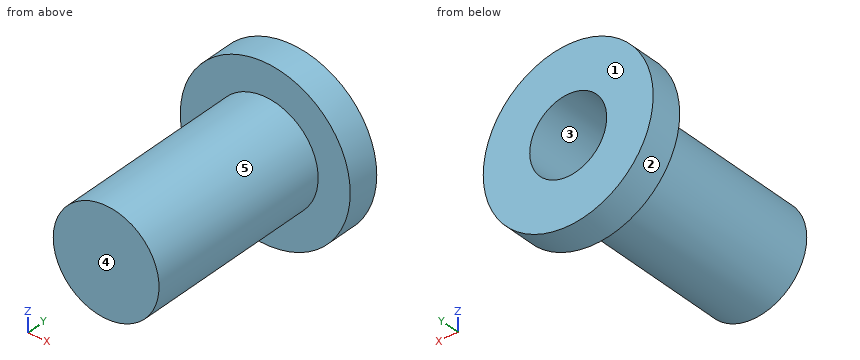
from build123d import *

# Parameters (mm, degrees)
SKETCH3_R          = 1.2
CUT_EXTRUDE1_DEPTH = 5.8


with BuildPart() as part:
    # Sketch2 → Revolve2 (revolve)
    with BuildSketch(Plane.XY):
        Polygon((-1.65, 0), (-1.65, -6), (0, -6), (0, 1), (-2.65, 1), (-2.65, 0), align=None)
    revolve(axis=Axis((0, 2, 0), (0, -1, 0)))

    # Sketch3 → Cut-Extrude1 (cut)
    with BuildSketch(Plane(origin=(0, 1, 0), x_dir=(1, 0, 0), z_dir=(0, 1, 0))):
        Circle(SKETCH3_R)
    extrude(amount=-CUT_EXTRUDE1_DEPTH, mode=Mode.SUBTRACT)


solid = part.part
Build history of the part. All positions in model axes, mm. Face numbers are marked on the shaded views. A direction names the side the tool comes from. Give positions to 0.01 mm unless a question says otherwise; leave off trailing zeros. Loops run counter-clockwise (first coordinate to the right, second up) from the corner with the lowest first, then second, coordinate; pieces in that order, holes last. Notation, with made-up numbers: (-23, 86.25) - (-10, 86.25) arc R19 ccw to (-10, 115.25) - close; hole circle Ø6 at (-25.75, 15.5). An arc over 180 degrees is marked (long way). Write item = value, one per line. Start each with the question number.
1) Band-saw the part on D-D on y = -5. Give the cut face in (x, z), plus the area to 3 significant figures.
2) Band-saw the part on C-C on y = -3.75. Give the cut face in (x, z).
3) Probe probe 1 along Z at (x, y) = (0, -2.7); probe 2 along Y at (x, z) = (-0.1, 0.7). List the from-to ranges inside material, lowest first. Write a range as from..to.
4) Drop flat-ended pins along their axis: pin 1 Ø1.5 at (x, y) = (0, -1) entering from +Z; pin 2 Ø1.5 at (x, y) = (1, -1.5) entering from -Z; pin 3 Ø1.9 at (x, z) = (0, 0) entering from +Y. Give the stop position or say it passes through.
5) Band-saw the part on B-B on x = 0. Give the cut face in (y, z), plus the area to 3 significant figures.
6) Band-saw the part on A-A on z = 0. Give the cut face in (x, y).
7) Tool access for the marked faces 4 and 5: list every direction of +Z, -Z, +X, -X, +Y, -Y with a clear straight run to the whole face (end or side of a thin tool).
8) Pull direction X, two halves, no side cores. Call the marked faces 1, 2 and 3: +X half, -X half, draft (parallel to the pull), parting line (faces both ways), or undercut.
Final values:
q1.outline = circle Ø3.3 at (0, 0)
q1.area = 8.55 mm²
q2.outline = circle Ø3.3 at (0, 0); hole circle Ø2.4 at (0, 0)
q3.probe_1 = -1.65..-1.2, 1.2..1.65
q3.probe_2 = -6..-4.8
q4.pin_1 = 1.65
q4.pin_2 = -1.63
q4.pin_3 = -4.8
q5.outline = (-6, -1.65) - (0, -1.65) - (0, -2.65) - (1, -2.65) - (1, -1.2) - (-4.8, -1.2) - (-4.8, 1.2) - (1, 1.2) - (1, 2.65) - (0, 2.65) - (0, 1.65) - (-6, 1.65) - close
q5.area = 11.2 mm²
q6.outline = (-2.65, 0) - (-1.65, 0) - (-1.65, -6) - (1.65, -6) - (1.65, 0) - (2.65, 0) - (2.65, 1) - (1.2, 1) - (1.2, -4.8) - (-1.2, -4.8) - (-1.2, 1) - (-2.65, 1) - close
q7.face_4 = +Z, -Z, +X, -X, -Y
q7.face_5 = -Y
q8.face_1 = draft
q8.face_2 = parting line
q8.face_3 = undercut
